```python
from build123d import *

# Parameters (mm, degrees)
BOSS_EXTRUDE1_DEPTH = 8.89
SKETCH2_R           = 2.032
CUT_EXTRUDE1_DEPTH  = 54.189709887
CUT_EXTRUDE2_REACH  = 55.452
SKETCH3_R           = 2.032
FILLET1_R           = 2.54
FILLET2_R           = 5.08
FILLET3_R           = 11.43
CHAMFER1_SIZE       = 0.635


with BuildPart() as part:
    # Sketch1 → Boss-Extrude1 (new body)
    with BuildSketch(Plane(origin=(0, 0, 0), x_dir=(1, 0, 0), z_dir=(0, 1, 0))):
        Polygon((3.81, -0.501596016), (3.81, -50.8), (-3.81, -50.8), (-3.81, 0.501596016), (9.467830093, 50.055132537), (16.828184889, 48.082931414), align=None)
    extrude(amount=BOSS_EXTRUDE1_DEPTH)

    # Sketch2 → Cut-Extrude1 (cut, through all)
    with BuildSketch(Plane(origin=(3.81, 0, 0), x_dir=(0, 0, -1), z_dir=(1, 0, 0))):
        with Locations((-40.833442343, 4.445)):
            Circle(SKETCH2_R)
        with Locations((-9.083442343, 4.445)):
            Circle(SKETCH2_R)
    extrude(amount=-CUT_EXTRUDE1_DEPTH, mode=Mode.SUBTRACT)

    # Sketch3 → Cut-Extrude2 (cut, up to next)
    with BuildSketch(Plane(origin=(3.680177398, 0, 0.986100562), x_dir=(0.25881904510251424, 0, -0.9659258262890701), z_dir=(0.9659258262890701, 0, 0.25881904510251424)), mode=Mode.PRIVATE) as cut_extrude2_sk1:
        with Locations((43.373442343, 4.445)):
            Circle(SKETCH3_R)
    cut_extrude2_tool1 = extrude(cut_extrude2_sk1.sketch, amount=-CUT_EXTRUDE2_REACH, mode=Mode.PRIVATE) & part.part
    # Sketch3 → Cut-Extrude2 (cut, up to next)
    with BuildSketch(Plane(origin=(3.680177398, 0, 0.986100562), x_dir=(0.25881904510251424, 0, -0.9659258262890701), z_dir=(0.9659258262890701, 0, 0.25881904510251424)), mode=Mode.PRIVATE) as cut_extrude2_sk2:
        with Locations((11.623442343, 4.445)):
            Circle(SKETCH3_R)
    cut_extrude2_tool2 = extrude(cut_extrude2_sk2.sketch, amount=-CUT_EXTRUDE2_REACH, mode=Mode.PRIVATE) & part.part
    add(cut_extrude2_tool1.solids().sort_by_distance((14.90605, 4.445, -40.909428))[0], mode=Mode.SUBTRACT)
    add(cut_extrude2_tool2.solids().sort_by_distance((6.688546, 4.445, -10.241283))[0], mode=Mode.SUBTRACT)

    # Fillet1
    fillet1_edges = [part.edges().sort_by_distance(p)[0] for p in [
        (13.148007491, 8.89, -49.069031975),
        (13.148007491, 0, -49.069031975),
        (0, 0, 50.8),
        (0, 8.89, 50.8),
    ]]
    fillet(fillet1_edges, radius=FILLET1_R)

    # Fillet2
    fillet2_edges = [part.edges().sort_by_distance(p)[0] for p in [
        (3.81, 4.445, 0.501596016),
    ]]
    fillet(fillet2_edges, radius=FILLET2_R)

    # Fillet3
    fillet3_edges = [part.edges().sort_by_distance(p)[0] for p in [
        (-3.81, 4.445, -0.501596016),
    ]]
    fillet(fillet3_edges, radius=FILLET3_R)

    # Chamfer1
    chamfer1_edges = [part.edges().sort_by_distance(p)[0] for p in [
        (-3.81, 4.445, 11.115442343),
        (3.81, 4.445, 11.115442343),
        (-3.81, 4.445, 42.865442343),
        (3.81, 4.445, 42.865442343),
        (-1.19772945, 4.445, -10.250722432),
        (6.162625347, 4.445, -8.278521309),
        (7.019775232, 4.445, -40.918867417),
        (14.380130029, 4.445, -38.946666293),
        (9.467830093, 4.445, -50.055132537),
        (16.828184889, 4.445, -48.082931414),
        (9.275281981, 8.146051224, -49.336533201),
        (9.275281981, 0.743948776, -49.336533201),
        (16.635636778, 8.146051224, -47.364332078),
        (16.635636778, 0.743948776, -47.364332078),
        (-3.81, 4.445, 50.8),
        (-3.81, 8.146051224, 50.056051224),
        (-3.81, 0.743948776, 50.056051224),
        (3.81, 4.445, 50.8),
        (3.81, 8.146051224, 50.056051224),
        (3.81, 0.743948776, 50.056051224),
        (10.076940659, 0, -22.88694493),
        (10.076940659, 8.89, -22.88694493),
        (3.81, 0, 24.715195352),
        (3.81, 8.89, 24.715195352),
        (3.853460104, 0, 0.507317647),
        (3.853460104, 8.89, 0.507317647),
        (-3.81, 0, 24.631596016),
        (-3.81, 8.89, 24.631596016),
        (2.694948762, 0, -24.778395296),
        (-3.712214766, 0, -0.488722345),
        (2.694948762, 8.89, -24.778395296),
        (-3.712214766, 8.89, -0.488722345),
    ]]
    chamfer(chamfer1_edges, length=CHAMFER1_SIZE)


solid = part.part
```
Work out the finished part from the listing and answer in its coordinate system (mm). A direction names the side the tool comes from. Round coordinates to 2 decimals unless told otherwise and drop trailing zeros. Loops run counter-clockwise (first coordinate to the right, second up) from the corner with the lowest first, then second, coordinate; pieces in that order, holes last. Notation, with made-up numbers: M 6,-11 L 56,-11 A25 cw 56,25 Z; hole C -4,-5.75 d11. An arc over 180 degrees is marked long. One line per question, with ' | ' between items.
Q1. Each of these flat-tipped pins is pushed along its axis until it touches: pin 1 Ø4.5 at (y, z) = (4.44, 40.83) entering from +X; pin 2 Ø1.5 at (y, z) = (4.5, 38.5) entering from +X; pin 3 Ø5 at (x, z) = (4.5, 32) entering from -Y. Where does it stop, or does it pass through?
Conclusion:
pin 1: stops at x = 3.4 | pin 2: stops at x = 3.81 | pin 3: stops at y = 0
Q2. Find section A-A, the plane z = 14.5. Give the vertices of the cut face in (x, y) (3 decimals), then the cut area to 3 significant figures.
Conclusion:
outline: M -3.81,0.635 L -3.175,0 L 3.175,0 L 3.81,0.635 L 3.81,8.255 L 3.175,8.89 L -3.175,8.89 L -3.81,8.255 Z | area: 66.9 mm2
Q3. Find section B-B, the plane z = -37.5. Give the vertices of the cut face in (x, y) (1 decimal).
Conclusion:
outline: M 6.1,0.6 L 6.8,0 L 13.3,0 L 14,0.6 L 14,8.3 L 13.3,8.9 L 6.8,8.9 L 6.1,8.3 Z
Q4. A tool of negligible diameter and unlimited length cuts with its end or side. For faces 4 (the cylindrical face through (0, 8.2, 50)), 5 (the flat face through (3.81, 4, 25)), from which of +Z, -Z, +X, -X, +Y, -Y can it reach the whole face along a straight path? Write none if from no direction.
Conclusion:
face 4: +Z, +X, -X, +Y | face 5: +Z, +X, +Y, -Y
Q5. The mould has two halves that part along Z. Classify faces 1 (the flat face through (2.92, 0.313, -24.376)), 2 (the conical face through (3.63, 1.08, 49.75)), 3 (the cylindrical face through (2.94, 2.46, -10.79)): +Z half, -Z half, draft (parallel to the pull), parting line (faces both ways), or undercut.
Conclusion:
face 1: -Z half | face 2: +Z half | face 3: undercut
Q6. Consider line 1 along Y through (x, z) = (1.5, 41.5); line 2 along X through (y, z) = (4.25, 37); line 3 along Y through (x, z) = (2, 10). Determine where each line is inside the solid, lowest interval first. Write a range as from..to.
Conclusion:
line 1: y = 0..2.53, 6.36..8.89 | line 2: x = -3.81..3.81 | line 3: y = 0..2.63, 6.26..8.89
